Source: three-view drawing plus pictorial views. Frame: mm from the lowest corner of the part. Coordinates: 2 decimals unless noted, no trailing zeros. Order: outer loops, then holes, each group sorted by start corner. A loop starts at its lowest first (then second) coordinate and runs counter-clockwise, first axis right, second up. Notation, with made-up numbers: (-19, 74.5) - (29, 74.5) arc R21 ccw to (29, 110.5) - close; hole circle Ø1 at (29.25, 78.25). An arc over 180 degrees is marked (long way). One line per question, with ' | ' between items.
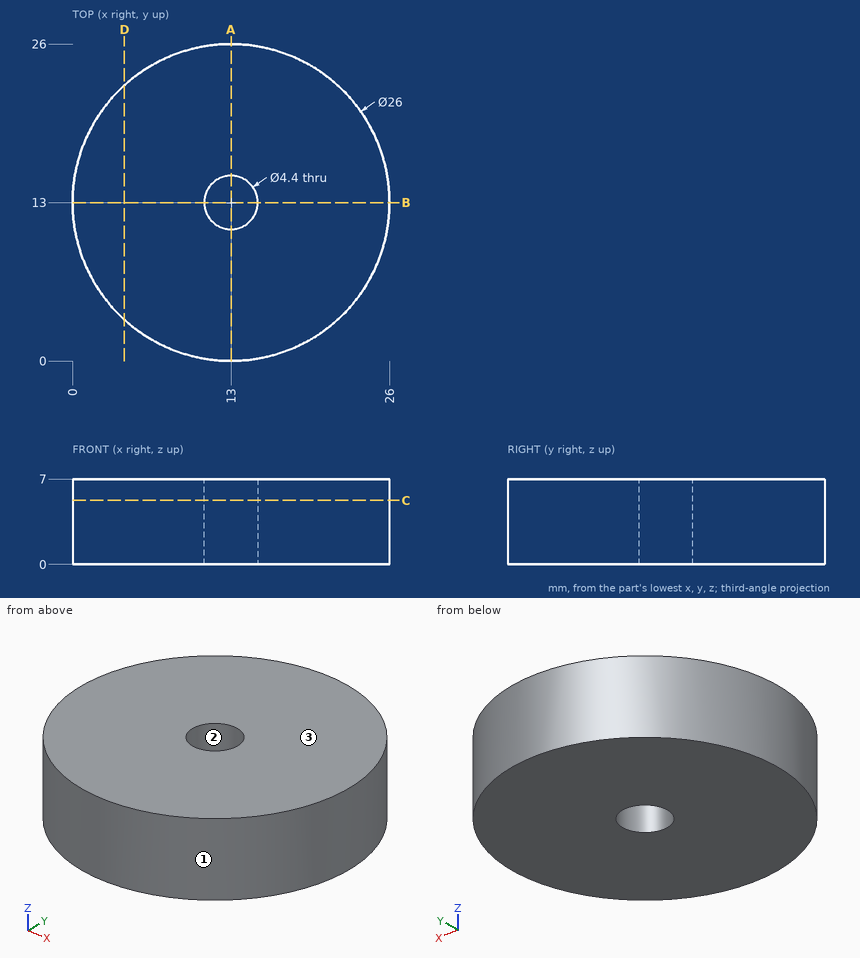
Item 1: Section C-C on z = 5.25. Return the cut outline in (x, y).
Data:
outline: circle Ø26 at (13, 13); hole circle Ø4.4 at (13, 13)
Item 2: Contact query for flat-ended pins moving along their axis: P1, Ø2, axis at y = 11.5, z = 2, coming from the +X side; P2, Ø1.5, axis at y = 15, z = 5, coming from the +X side; P3, Ø2, axis at y = 11, z = 3, coming from the -X side. Output: stop coordinate, or through.
Data:
P1: x = 25.99 | P2: x = 25.94 | P3: x = 0.04
Item 3: Ray query, line 1 (Y direction, x = 13, z = 5); line 2 (Y direction, x = 15, z = 5.5); line 3 (X direction, y = 12.75, z = 6.25). Return the intervals inside material, ascending.
Data:
line 1: 0 to 10.8, 15.2 to 26 | line 2: 0.15 to 12.08, 13.92 to 25.85 | line 3: 0 to 10.81, 15.19 to 26
Item 4: Section D-D on x = 4.25. Return the cut outline in (y, z), and give its area (3 significant figures).
Data:
outline: (3.39, 0) - (22.61, 0) - (22.61, 7) - (3.39, 7) - close | area: 135 mm^2
Item 5: Section A-A on x = 13. Return the cut outline in (y, z), and give its area (3 significant figures).
Data:
outline: (0, 0) - (10.8, 0) - (10.8, 7) - (0, 7) - close; (15.2, 0) - (26, 0) - (26, 7) - (15.2, 7) - close | area: 151 mm^2
Item 6: Draft query along X for the marked faces 1, 2 and 3. Return one class per face: released by +X, released by -X, zero draft, split by the parting line, or undercut.
Data:
face 1: split by the parting line | face 2: undercut | face 3: zero draft
